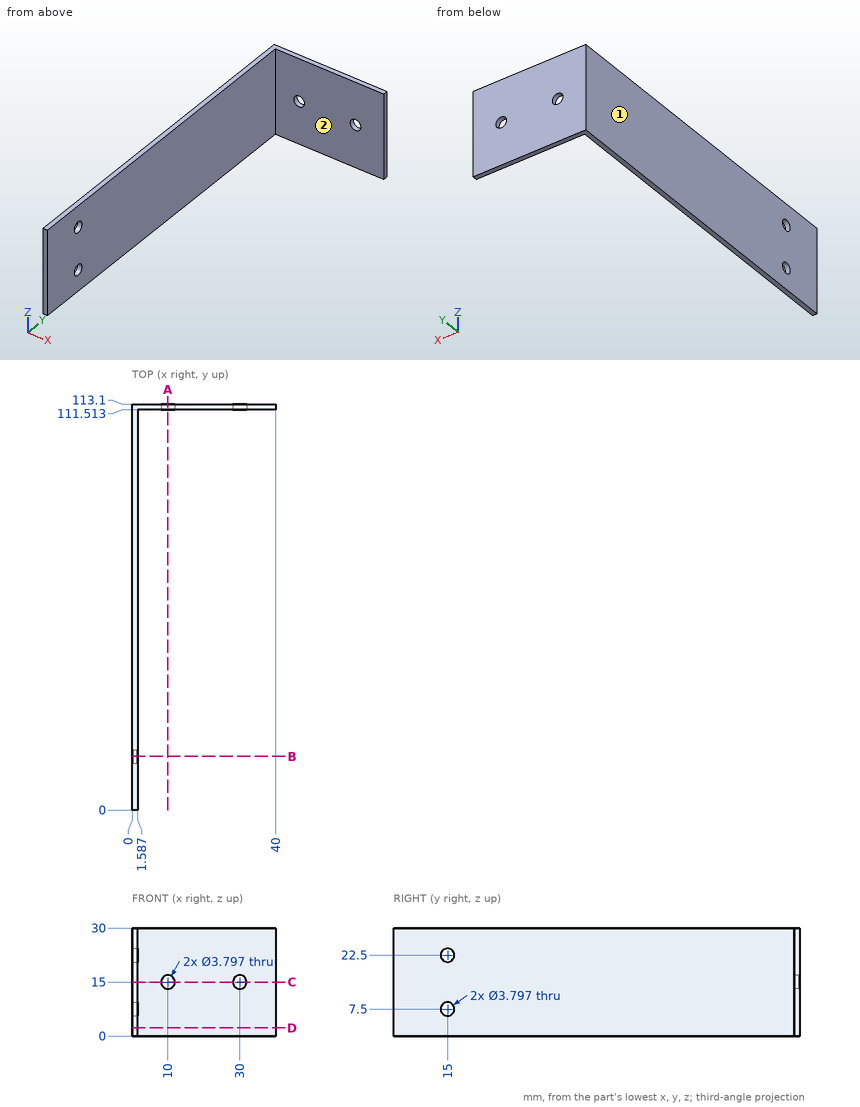
Geometry check sheet. Reference: drawing and pictorial views, mm from the part's lowest x, y, z. A direction names the side the tool comes from. Coordinates: 2 decimals unless noted, no trailing zeros. Order: outer loops, then holes, each group sorted by start corner. A loop starts at its lowest first (then second) coordinate and runs counter-clockwise, first axis right, second up. Notation, with made-up numbers: (72.25, 82) -> (76.25, 82) arc R21 ccw to (76.25, 100) -> close; hole circle Ø6 at (67, 89.25). An arc over 180 degrees is marked (long way). Use CSV: the item, a comma, the result in double quotes. Start each with the question number.
Q1. Depth check by flat-ended pin: P1, Ø4, axis at x = 15, z = 12.5, coming from the -Y side; P2, Ø10, axis at y = 35.5, z = 22.5, coming from the +X side; P3, Ø3.5, axis at y = 15, z = 22.5, coming from the -X side. Enter the tip coordinate at first touch or a pass-through.
Q2. Section check D-D, the plane z = 2.25. Record the cut outline in (x, y).
Q3. Section check A-A, the plane x = 10. Record the cut outline in (y, z).
Q4. Thickness scan on line 1 along X through (y, z) = (112.3, 15); line 2 along Y through (x, z) = (0.4, 22.5); line 3 along X through (y, z) = (47.5, 13.5). Record the ranges inside material, lowest first.
Q5. Section check B-B, the plane y = 15. Record the cut outline in (x, z).
Q6. Tool access check on the marked faces 1 and 2. Record the directions out of +Z, -Z, +X, -X, +Y, -Y that give a thin tool (end or side, any length) a straight path to the whole face; none if there is none.
Q7. Section check C-C, the plane z = 15. Record the cut outline in (x, y).
Returned:
1,P1,"stops at y = 111.51"
1,P2,"stops at x = 1.59"
1,P3,"passes through"
2,outline,"(0, 0) -> (1.59, 0) -> (1.59, 111.51) -> (40, 111.51) -> (40, 113.1) -> (0, 113.1) -> close"
3,outline,"(111.51, 0) -> (113.1, 0) -> (113.1, 13.1) -> (111.51, 13.1) -> close; (111.51, 16.9) -> (113.1, 16.9) -> (113.1, 30) -> (111.51, 30) -> close"
4,line 1,"x = 0 to 8.1, 11.9 to 28.1, 31.9 to 40"
4,line 2,"y = 0 to 13.1, 16.9 to 113.1"
4,line 3,"x = 0 to 1.59"
5,outline,"(0, 0) -> (1.59, 0) -> (1.59, 5.6) -> (0, 5.6) -> close; (0, 9.4) -> (1.59, 9.4) -> (1.59, 20.6) -> (0, 20.6) -> close; (0, 24.4) -> (1.59, 24.4) -> (1.59, 30) -> (0, 30) -> close"
6,face 1,"+Z, -Z, -X, +Y, -Y"
6,face 2,"+Z, -Z, +X, -Y"
7,outline,"(0, 0) -> (1.59, 0) -> (1.59, 111.51) -> (8.1, 111.51) -> (8.1, 113.1) -> (0, 113.1) -> close; (11.9, 111.51) -> (28.1, 111.51) -> (28.1, 113.1) -> (11.9, 113.1) -> close; (31.9, 111.51) -> (40, 111.51) -> (40, 113.1) -> (31.9, 113.1) -> close"
